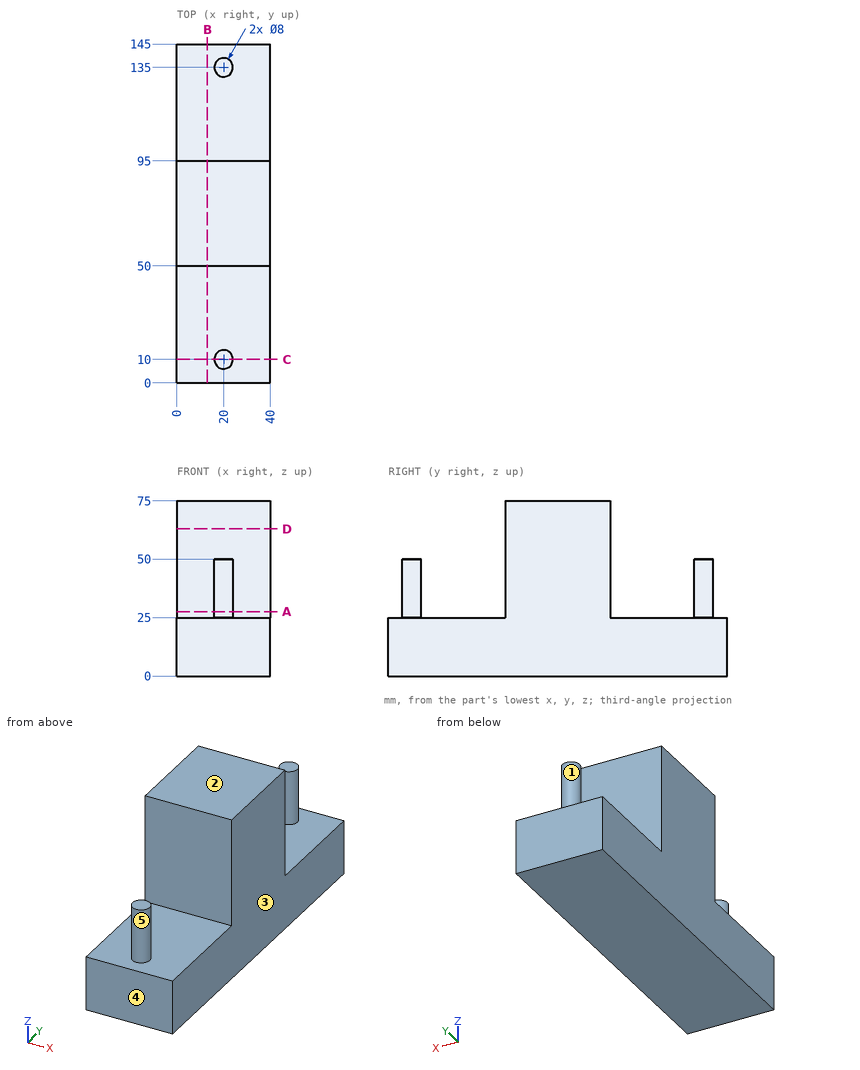
Drawing for the job (mm, zero at the part's lowest x, y, z). A direction names the side the tool comes from. Coordinates: 2 decimals unless noted, no trailing zeros. Order: outer loops, then holes, each group sorted by start corner. A loop starts at its lowest first (then second) coordinate and runs counter-clockwise, first axis right, second up. Notation, with made-up numbers: (-11.5, 55) - (44.5, 55) arc R8 cw to (44.5, 70) - close; hole circle Ø11 at (76.25, -4). An arc over 180 degrees is marked (long way). Use a Markdown table: item, result. Add a question column.
(1) Saw through at A-A (z = 27.5). Give the cut face in (x, y), then the cut area to 3 significant figures.
(2) Flat gauge pins, fed straight in: pin 1 (4 mm diameter, centred on x = 33.5, y = 14.5, fed in from +Z); pin 2 (8 mm diameter, centred on x = 28.5, z = 34, fed in from -Y); pin 3 (6.5 mm diameter, centred on x = 18.5, y = 136, fed in from +Z). Where does each tip first touch, or does it go through?
(3) Pull direction Y, two halves, no side cores. Call the marked faces 3, 4 and 5: +Y half, -Y half, draft (parallel to the pull), parting line (faces both ways), or undercut.
(4) Which spindle directions (+Z, -Z, +X, -X, +Y, -Y) get a long thin tool onto all of the face, cutting with end or side? Do the marked faces 1 and 2. Say none if no direction does.
(5) Saw through at C-C (y = 10). Give the cut face in (x, z).
(6) Saw through at D-D (z = 63). Give the cut face in (x, y), then the cut area to 3 significant figures.
(7) Drill centre lines: line 1 along Y through (x, z) = (27.5, 56); line 2 along Z through (x, y) = (23, 128.5); line 3 along X through (y, z) = (134.5, 40). Where is each one in solid material? Low to high. Write a range as [from, to].
(8) Saw through at B-B (x = 13). Give the cut face in (y, z).
Solved:
| question | item | result |
|---|---|---|
| 1 | outline | (0, 50) - (40, 50) - (40, 95) - (0, 95) - close; circle Ø8 at (20, 10); circle Ø8 at (20, 135) |
| 1 | area | 1,900 mm² |
| 2 | pin 1 | stops at z = 25 |
| 2 | pin 2 | stops at y = 50 |
| 2 | pin 3 | stops at z = 50 |
| 3 | face 3 | draft |
| 3 | face 4 | -Y half |
| 3 | face 5 | undercut |
| 4 | face 1 | +Z |
| 4 | face 2 | +Z, +X, -X, +Y, -Y |
| 5 | outline | (0, 0) - (40, 0) - (40, 25) - (24, 25) - (24, 50) - (16, 50) - (16, 25) - (0, 25) - close |
| 6 | outline | (0, 50) - (40, 50) - (40, 95) - (0, 95) - close |
| 6 | area | 1,800 mm² |
| 7 | line 1 | y = [50, 95] |
| 7 | line 2 | z = [0, 25] |
| 7 | line 3 | x = [16.03, 23.97] |
| 8 | outline | (0, 0) - (145, 0) - (145, 25) - (95, 25) - (95, 75) - (50, 75) - (50, 25) - (0, 25) - close |
